from build123d import *

# Parameters (mm, degrees)
SKETCH2_R          = 1.75
CUT_EXTRUDE1_DEPTH = 10
CUT_EXTRUDE2_DEPTH = 15
CUT_EXTRUDE3_START = -10
CUT_EXTRUDE3_DEPTH = 10


with BuildPart() as part:
    # Sketch1 → Revolve1 (revolve)
    with BuildSketch(Plane(origin=(0, 0, 0), x_dir=(0, 0, -1), z_dir=(1, 0, 0))):
        Polygon((-5.25, 80), (-5.25, -60), (-25, -60), (-25, -65), (-10, -65), (-10, -80), (0, -80), (0, 80), align=None)
    revolve(axis=Axis((0, 49.914529915, 0), (0, -1, 0)))

    # Sketch2 → Cut-Extrude1 (cut)
    with BuildSketch(Plane(origin=(0, -60, 0), x_dir=(1, 0, 0), z_dir=(0, 1, 0))):
        with Locations(Location((0, -21.25, 0), (0, 0, 270))):
            Circle(SKETCH2_R)
        with Locations(Location((-15.0260191, -15.0260191, 0), (0, 0, 270))):
            Circle(SKETCH2_R)
        with Locations(Location((-21.25, 0, 0), (0, 0, 270))):
            Circle(SKETCH2_R)
        with Locations(Location((-15.0260191, 15.0260191, 0), (0, 0, 270))):
            Circle(SKETCH2_R)
        with Locations(Location((0, 21.25, 0), (0, 0, 270))):
            Circle(SKETCH2_R)
        with Locations(Location((15.0260191, 15.0260191, 0), (0, 0, 270))):
            Circle(SKETCH2_R)
        with Locations(Location((21.25, 0, 0), (0, 0, 270))):
            Circle(SKETCH2_R)
        with Locations(Location((15.0260191, -15.0260191, 0), (0, 0, 270))):
            Circle(SKETCH2_R)
    extrude(amount=-CUT_EXTRUDE1_DEPTH, mode=Mode.SUBTRACT)

    # Sketch3 → Cut-Extrude2 (cut)
    with BuildSketch(Plane.XZ.offset(80)):
        with BuildLine():
            Line((-3, 9.539392014), (-3, 3))
            Line((-3, 3), (-9.539392014, 3))
            ThreePointArc((-9.539392014, 3), (-7.071067812, 7.071067812), (-3, 9.539392014))
        make_face()
        with BuildLine():
            Line((-3, -3), (-9.539392014, -3))
            ThreePointArc((-9.539392014, -3), (-7.071067812, -7.071067812), (-3, -9.539392014))
            Line((-3, -9.539392014), (-3, -3))
        make_face()
        with BuildLine():
            Line((3, -3), (9.539392014, -3))
            ThreePointArc((9.539392014, -3), (7.071067812, -7.071067812), (3, -9.539392014))
            Line((3, -9.539392014), (3, -3))
        make_face()
        with BuildLine():
            Line((3, 3), (9.539392014, 3))
            ThreePointArc((9.539392014, 3), (7.071067812, 7.071067812), (3, 9.539392014))
            Line((3, 9.539392014), (3, 3))
        make_face()
    extrude(amount=-CUT_EXTRUDE2_DEPTH, mode=Mode.SUBTRACT)

    # Sketch4 → Cut-Extrude3 (cut)
    with BuildSketch(Plane(origin=(0, 80, 0), x_dir=(1, 0, 0), z_dir=(0, 1, 0)).offset(CUT_EXTRUDE3_START)):
        with BuildLine():
            Line((-1.5, -1.5), (-5.031152949, -1.5))
            ThreePointArc((-5.031152949, -1.5), (-3.712310601, -3.712310601), (-1.5, -5.031152949))
            Line((-1.5, -5.031152949), (-1.5, -1.5))
        make_face()
        with BuildLine():
            Line((1.5, -1.5), (1.5, -5.031152949))
            ThreePointArc((1.5, -5.031152949), (3.712310601, -3.712310601), (5.031152949, -1.5))
            Line((5.031152949, -1.5), (1.5, -1.5))
        make_face()
        with BuildLine():
            ThreePointArc((5.031152949, 1.5), (3.712310601, 3.712310601), (1.5, 5.031152949))
            Line((1.5, 5.031152949), (1.5, 1.5))
            Line((1.5, 1.5), (5.031152949, 1.5))
        make_face()
        with BuildLine():
            ThreePointArc((-5.031152949, 1.5), (-3.712310601, 3.712310601), (-1.5, 5.031152949))
            Line((-1.5, 5.031152949), (-1.5, 1.5))
            Line((-1.5, 1.5), (-5.031152949, 1.5))
        make_face()
    extrude(amount=CUT_EXTRUDE3_DEPTH, mode=Mode.SUBTRACT)


solid = part.part
Geometry: final body of the model. Coordinates: model frame, mm. A direction names the side the tool comes from. Coordinates: 2 decimals unless noted, no trailing zeros. Order: outer loops, then holes, each group sorted by start corner. A loop starts at its lowest first (then second) coordinate and runs counter-clockwise, first axis right, second up.
(1) Section query A-A (z = 0). Return the cut outline in (x, y).
(2) First-contact query: pin 1 (3.5 mm diameter, centred on x = -6.5, y = -71, fed in from +Z); pin 2 (3 mm diameter, centred on y = 74, z = -3.5, fed in from +X); pin 3 (5 mm diameter, centred on x = -5, y = -75, fed in from -Z); pin 4 (2 mm diameter, centred on x = 0, z = 21.25, fed in from +Y). Flat tips, straight axial feed; report the tip coordinate or a pass-through.
(3) Access query for faces 1 (the face through (-3, -73, -6)), 2 (the face through (1.5, 75, 3)), 3 (the face through (-3, 70, -3)), 4 (the face through (3, 75, -1.5)), 5 (the face through (-3, 70, 3)). Directions: +Z, -Z, +X, -X, +Y, -Y. A direction counts if a zero-diameter tool reaches every point of the face in a straight line with its end or side. Return the directions, or none.
(4) Section query C-C (z = -21.25). Return the cut outline in (x, y).
(5) Section query D-D (x = 21.25). Return the cut outline in (y, z).
(6) Material intervals for probe 1 along X at (y, z) = (-61.35, 0); probe 2 along Y at (x, z) = (19.5, 3); probe 3 along Z at (x, y) = (21, -63), sorted ascending.
(7) Draft query along Z for faces 6 (the face through (-1.5, 75, -3)), 7 (the face through (16.76, -62.46, 14.8)), 8 (the face through (-10, -73, 0)), 9 (the face through (16.502, -62.465, -14.085)). Return one class per face: pulls with the +Z half, pulls with the -Z half, needs draft (parallel to the pull), parting line crosses it, or undercut.
(8) Section query B-B (x = 0). Return the cut outline in (y, z).
Solution:
1. outline: (-25, -65) - (-23, -65) - (-23, -60) - (-25, -60) - close; (-19.5, -65) - (-10, -65) - (-10, -80) - (10, -80) - (10, -65) - (19.5, -65) - (19.5, -60) - (5.25, -60) - (5.25, 80) - (-5.25, 80) - (-5.25, -60) - (-19.5, -60) - close; (23, -65) - (25, -65) - (25, -60) - (23, -60) - close
2. pin 1: stops at z = 3
2. pin 2: stops at x = 1.5
2. pin 3: stops at z = -9.68
2. pin 4: passes through
3. face 1: -Z, -X, -Y
3. face 2: +Z, +X, +Y
3. face 3: -Z, -X, +Y
3. face 4: -Z, +X, +Y
3. face 5: +Z, -X, +Y
4. outline: (-13.17, -65) - (-1.75, -65) - (-1.75, -60) - (-13.17, -60) - close; (1.75, -65) - (13.17, -65) - (13.17, -60) - (1.75, -60) - close
5. outline: (-65, -13.17) - (-60, -13.17) - (-60, -1.75) - (-65, -1.75) - close; (-65, 1.75) - (-60, 1.75) - (-60, 13.17) - (-65, 13.17) - close
6. probe 1: x = -25 to -23, -19.5 to 19.5, 23 to 25
6. probe 2: y = -65 to -60
6. probe 3: z = -13.56 to -1.73, 1.73 to 13.56
7. face 6: needs draft
7. face 7: undercut
7. face 8: parting line crosses it
7. face 9: undercut
8. outline: (-80, -10) - (-65, -10) - (-65, -19.5) - (-60, -19.5) - (-60, -5.25) - (80, -5.25) - (80, 5.25) - (-60, 5.25) - (-60, 19.5) - (-65, 19.5) - (-65, 10) - (-80, 10) - close; (-65, -25) - (-60, -25) - (-60, -23) - (-65, -23) - close; (-65, 23) - (-60, 23) - (-60, 25) - (-65, 25) - close
